Source: CAD feature listing. Evaluate the final solid. Frame: model axes, mm. A direction names the side the tool comes from. Coordinates: 2 decimals unless noted, no trailing zeros. Write each loop counter-clockwise with the first axis right and the second up, starting at its lowest first coordinate (ties: lowest second). Pieces come first, ordered by that corner, then holes. Notation, with made-up numbers: M 17,-30.75 L 54,-30.75 A10 ccw 54,-25.75 Z; hole C -33.75,14 d8. An arc over 180 degrees is marked long. Answer as CSV lines item,"result". Start each with the question number.
1. Contact query for flat-ended pins moving along their axis: pin 1 Ø4 at (x, y) = (-3.5, -1) entering from +Z; pin 2 Ø1.5 at (x, y) = (18.5, -13) entering from -Z; pin 3 Ø4 at (y, z) = (-18, 24) entering from +X. Output: stop coordinate, or through.
2. Mould query, pull axis Y, two halves, no side actions, for faces 4 (the face through (-0.78, -9.99, 34.58)), 5 (the face through (7.81, -1.73, -7.44)), 6 (the face through (-9, 1, 0)). Classes: pulls with the +Y half, pulls with the -Y half, needs draft (parallel to the pull), parting line crosses it, or undercut.
3. Reachability of faces 1 (the face through (0, -6, -22)), 2 (the face through (0, -16, 5)), 3 (the face through (0, 0, -30)) from +Z, -Z, +X, -X, +Y, -Y: full face, straight path, thin tool, end or side. Return the list, or none.
4. Section B-B on x = 0. Return the cut outline in (y, z), plus the area to 3 significant figures.
5. Line query: probe 1 along Y at (x, z) = (0, 20); probe 2 along X at (y, z) = (-16, 18.5); probe 3 along Z at (x, y) = (19.5, 11). Output: solid intervals per line, ascending. Write a range as [from, to].
6. Section C-C on z = -18.5. Return the cut outline in (x, y).
7. Section A-A on y = 0. Return the cut outline in (x, z), plus the area to 3 significant figures.
```python
from build123d import *

# Parameters (mm, degrees)
SKETCH2_R           = 9.525
SKETCH2_R_2         = 6
BOSS_EXTRUDE1_DEPTH = 60


with BuildPart() as part:
    # Sketch1 → Revolve1 (revolve)
    with BuildSketch(Plane(origin=(0, 0, 0), x_dir=(0, 0, -1), z_dir=(1, 0, 0))):
        Polygon((0, 8), (0, 37.25), (-5, 37.25), (-5, 0), (30, 0), (30, 6), (15.1, 6), (15.1, 8), align=None)
    revolve(axis=Axis((0, 0, -30), (0, 0, 1)))

    # Sketch2 → Boss-Extrude1 (add)
    with BuildSketch(Plane.XY.offset(5)):
        with Locations((0, -15.9375)):
            Circle(SKETCH2_R)
        with Locations((0, -15.9375)):
            Circle(SKETCH2_R_2, mode=Mode.SUBTRACT)
    extrude(amount=BOSS_EXTRUDE1_DEPTH)


solid = part.part
```
Values:
1,pin 1,"z = 5"
1,pin 2,"z = 0"
1,pin 3,"x = 9.52"
2,face 4,"undercut"
2,face 5,"parting line crosses it"
2,face 6,"needs draft"
3,face 1,"-Z"
3,face 2,"+Z"
3,face 3,"-Z, +X, -X, +Y, -Y"
4,outline,"M -37.25,0 L -8,0 L -8,-15.1 L -6,-15.1 L -6,-30 L 6,-30 L 6,-15.1 L 8,-15.1 L 8,0 L 37.25,0 L 37.25,5 L -6.41,5 L -6.41,65 L -9.94,65 L -9.94,5 L -21.94,5 L -21.94,65 L -25.46,65 L -25.46,5 L -37.25,5 Z"
4,area,"1,220 mm²"
5,probe 1,"[-25.46, -21.94], [-9.94, -6.41]"
5,probe 2,"[-9.52, -6], [6, 9.52]"
5,probe 3,"[0, 5]"
6,outline,"C 0,0 d12"
7,outline,"M -37.25,0 L -8,0 L -8,-15.1 L -6,-15.1 L -6,-30 L 6,-30 L 6,-15.1 L 8,-15.1 L 8,0 L 37.25,0 L 37.25,5 L -37.25,5 Z"
7,area,"793 mm²"
